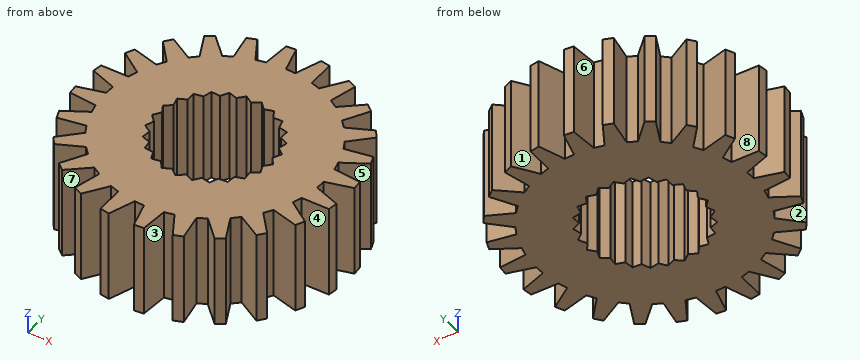
```python
from build123d import *

# Parameters (mm, degrees)
F1_DEPTH = 5.08


# Not quite as in the source:
# - ends of sketch curves that miss each other by under 0.0002 mm in the source are joined


with BuildPart() as f1:
    # F0 (on Top) → F1 (new body)
    with BuildSketch(Plane.XY):
        with BuildLine():
            Line((1.0386822, 7.3975722), (0.5233416, 5.9817))
            ThreePointArc((0.5233416, 5.9817), (0.261920534, 5.9988447577), (0, 6.00456))
            Line((0, 6.00456), (-0.3899662, 7.4599546))
            Line((-0.3899662, 7.4599546), (-0.911352, 7.4143362))
            Line((-0.911352, 7.4143362), (-1.04267, 5.9133486))
            ThreePointArc((-1.04267, 5.9133486), (-1.2996201412, 5.8622289517), (-1.5540978425, 5.79995868))
            Line((-1.5540978425, 5.79995868), (-2.307463, 7.1048372))
            Line((-2.307463, 7.1048372), (-2.7992832, 6.925818))
            Line((-2.7992832, 6.925818), (-2.5376378, 5.4419754))
            ThreePointArc((-2.5376378, 5.4419754), (-2.7726007409, 5.3261079528), (-3.0022844594, 5.2000989239))
            Line((-3.0022844594, 5.2000989239), (-4.0677084, 6.2655196))
            Line((-4.0677084, 6.2655196), (-4.496435, 5.965317))
            Line((-4.496435, 5.965317), (-3.859657, 4.5997622))
            ThreePointArc((-3.859657, 4.5997622), (-4.0566214385, 4.4270264624), (-4.245865094, 4.245865094))
            Line((-4.245865094, 4.245865094), (-5.5507382, 4.999228))
            Line((-5.5507382, 4.999228), (-5.8871612, 4.598289))
            Line((-5.8871612, 4.598289), (-4.9186338, 3.4440622))
            ThreePointArc((-4.9186338, 3.4440622), (-5.0641936548, 3.2262491255), (-5.2000989239, 3.0022844594))
            Line((-5.2000989239, 3.0022844594), (-6.6554858, 3.3922462))
            Line((-6.6554858, 3.3922462), (-6.876669, 2.9179012))
            Line((-6.876669, 2.9179012), (-5.6424322, 2.0536916))
            ThreePointArc((-5.6424322, 2.0536916), (-5.7266481207, 1.8056140494), (-5.79995868, 1.5540978425))
            Line((-5.79995868, 1.5540978425), (-7.306691, 1.554099))
            Line((-7.306691, 1.554099), (-7.3975722, 1.0386568))
            Line((-7.3975722, 1.0386568), (-5.9817, 0.5233416))
            ThreePointArc((-5.9817, 0.5233416), (-5.9988447577, 0.261920534), (-6.00456, 0))
            Line((-6.00456, 0), (-7.4599546, -0.3899662))
            Line((-7.4599546, -0.3899662), (-7.4143362, -0.911352))
            Line((-7.4143362, -0.911352), (-5.9133232, -1.04267))
            ThreePointArc((-5.9133232, -1.04267), (-5.8622284744, -1.2996222942), (-5.79995868, -1.5540978425))
            Line((-5.79995868, -1.5540978425), (-7.1048372, -2.307463))
            Line((-7.1048372, -2.307463), (-6.925818, -2.7992832))
            Line((-6.925818, -2.7992832), (-5.4419754, -2.5376378))
            ThreePointArc((-5.4419754, -2.5376378), (-5.3261079528, -2.7726007409), (-5.2000989239, -3.0022844594))
            Line((-5.2000989239, -3.0022844594), (-6.2655196, -4.0677084))
            Line((-6.2655196, -4.0677084), (-5.965317, -4.496435))
            Line((-5.965317, -4.496435), (-4.5997622, -3.859657))
            ThreePointArc((-4.5997622, -3.859657), (-4.4270264624, -4.0566214385), (-4.245865094, -4.245865094))
            Line((-4.245865094, -4.245865094), (-4.999228, -5.5507382))
            Line((-4.999228, -5.5507382), (-4.598289, -5.8871612))
            Line((-4.598289, -5.8871612), (-3.4440622, -4.9186592))
            ThreePointArc((-3.4440622, -4.9186592), (-3.2262429819, -5.0641975688), (-3.0022844594, -5.2000989239))
            Line((-3.0022844594, -5.2000989239), (-3.3922462, -6.6554858))
            Line((-3.3922462, -6.6554858), (-2.9179012, -6.8766944))
            Line((-2.9179012, -6.8766944), (-2.0536662, -5.6424322))
            ThreePointArc((-2.0536662, -5.6424322), (-1.8056026676, -5.7266517094), (-1.5540978425, -5.79995868))
            Line((-1.5540978425, -5.79995868), (-1.554099, -7.306691))
            Line((-1.554099, -7.306691), (-1.0386568, -7.3975722))
            Line((-1.0386568, -7.3975722), (-0.5233162, -5.9817))
            ThreePointArc((-0.5233162, -5.9817), (-0.2619078943, -5.9988453096), (0, -6.00456))
            Line((0, -6.00456), (0.3899662, -7.4599546))
            Line((0.3899662, -7.4599546), (0.9113774, -7.4143362))
            Line((0.9113774, -7.4143362), (1.0426954, -5.9133486))
            ThreePointArc((1.0426954, -5.9133486), (1.2996323518, -5.8622262447), (1.5540978425, -5.79995868))
            Line((1.5540978425, -5.79995868), (2.307463, -7.1048372))
            Line((2.307463, -7.1048372), (2.7992832, -6.925818))
            Line((2.7992832, -6.925818), (2.5376378, -5.4419754))
            ThreePointArc((2.5376378, -5.4419754), (2.7726007409, -5.3261079528), (3.0022844594, -5.2000989239))
            Line((3.0022844594, -5.2000989239), (4.0677084, -6.2655196))
            Line((4.0677084, -6.2655196), (4.496435, -5.965317))
            Line((4.496435, -5.965317), (3.859657, -4.5997622))
            ThreePointArc((3.859657, -4.5997622), (4.0566214385, -4.4270264624), (4.245865094, -4.245865094))
            Line((4.245865094, -4.245865094), (5.5507382, -4.999228))
            Line((5.5507382, -4.999228), (5.8871612, -4.598289))
            Line((5.8871612, -4.598289), (4.9186592, -3.4440622))
            ThreePointArc((4.9186592, -3.4440622), (5.0642009806, -3.2262376264), (5.2001052739, -3.0022734609))
            Line((5.2001052739, -3.0022734609), (6.6555112, -3.3922462))
            Line((6.6555112, -3.3922462), (6.8766944, -2.9179012))
            Line((6.8766944, -2.9179012), (5.6424576, -2.0536916))
            ThreePointArc((5.6424576, -2.0536916), (5.7266494269, -1.8056099067), (5.79995868, -1.5540978425))
            Line((5.79995868, -1.5540978425), (7.306691, -1.554099))
            Line((7.306691, -1.554099), (7.3975722, -1.0386568))
            Line((7.3975722, -1.0386568), (5.9817254, -0.5233416))
            ThreePointArc((5.9817254, -0.5233416), (5.998844806, -0.2619194281), (6.00456, 0))
            Line((6.00456, 0), (7.4599546, 0.3899662))
            Line((7.4599546, 0.3899662), (7.4143362, 0.911352))
            Line((7.4143362, 0.911352), (5.9133486, 1.04267))
            ThreePointArc((5.9133486, 1.04267), (5.8622289517, 1.2996201412), (5.79995868, 1.5540978425))
            Line((5.79995868, 1.5540978425), (7.1048372, 2.307463))
            Line((7.1048372, 2.307463), (6.925818, 2.7992832))
            Line((6.925818, 2.7992832), (5.4419754, 2.5376378))
            ThreePointArc((5.4419754, 2.5376378), (5.3261108849, 2.7725951084), (5.2001052739, 3.0022734609))
            Line((5.2001052739, 3.0022734609), (6.2655196, 4.0677084))
            Line((6.2655196, 4.0677084), (5.9653424, 4.496435))
            Line((5.9653424, 4.496435), (4.5997622, 3.859657))
            ThreePointArc((4.5997622, 3.859657), (4.4270264624, 4.0566214385), (4.245865094, 4.245865094))
            Line((4.245865094, 4.245865094), (4.999228, 5.5507382))
            Line((4.999228, 5.5507382), (4.5983144, 5.8871612))
            Line((4.5983144, 5.8871612), (3.4440876, 4.9186592))
            ThreePointArc((3.4440876, 4.9186592), (3.2262517559, 5.0641919791), (3.0022844594, 5.2000989239))
            Line((3.0022844594, 5.2000989239), (3.3922462, 6.6554858))
            Line((3.3922462, 6.6554858), (2.9179012, 6.8766944))
            Line((2.9179012, 6.8766944), (2.0536916, 5.6424322))
            ThreePointArc((2.0536916, 5.6424322), (1.8056140494, 5.7266481207), (1.5540978425, 5.79995868))
            Line((1.5540978425, 5.79995868), (1.554099, 7.306691))
            Line((1.554099, 7.306691), (1.0386822, 7.3975722))
        make_face()
        Polygon((-1.2318492, 3.1113222), (-0.7605522, 2.9622242), (-0.4194048, 3.319907), (0, 3.0583124), (0.4194048, 3.319907), (0.7605776, 2.9622242), (1.2318492, 3.1113222), (1.4733524, 2.6800048), (1.9668998, 2.7072082), (2.0935442, 2.2294088), (2.5783794, 2.1330158), (2.5822148, 1.6387318), (3.0278324, 1.4247876), (2.9086302, 0.9450578), (3.2870394, 0.6270244), (3.0522672, 0.192024), (3.3396936, -0.2101088), (3.0041342, -0.5730748), (3.1825184, -1.0340594), (2.7672284, -1.3021564), (2.825369, -1.7930368), (2.3564596, -1.9494246), (2.290699, -2.4393398), (1.7976342, -2.474214), (1.6120872, -2.9323792), (1.1258296, -2.84353), (0.8322056, -3.241167), (0.3833114, -3.0341824), (0, -3.3462976), (-0.3833114, -3.0341824), (-0.8321802, -3.241167), (-1.1258296, -2.84353), (-1.6120872, -2.9323792), (-1.7976088, -2.474214), (-2.290699, -2.4393398), (-2.3564596, -1.9494246), (-2.825369, -1.7930368), (-2.7672284, -1.3021564), (-3.1825184, -1.0340594), (-3.0041342, -0.5730748), (-3.3396936, -0.2101088), (-3.0522672, 0.192024), (-3.287014, 0.6270244), (-2.9086048, 0.9450578), (-3.027807, 1.4247876), (-2.5822148, 1.6387318), (-2.578354, 2.1330158), (-2.0935442, 2.2294088), (-1.9668998, 2.7072082), (-1.4733524, 2.6800048), align=None, mode=Mode.SUBTRACT)
    extrude(amount=F1_DEPTH)


solid = f1.part
```
Could you check a few things on this model? Use its own coordinates, in mm. Face numbers are marked on the shaded views. A direction names the side the tool comes from. Round coordinates to 2 decimals unless told otherwise and drop trailing zeros. Put each result on its own line as item: value.
Q1. Thinking about a two-plate mould opening in Y: for the marked faces 1, 2, 3 and 4, which applies, pulls with the +Y half, pulls with the -Y half, needs draft (parallel to the pull), parting line crosses it, or undercut?
Checks:
face 1: pulls with the +Y half
face 2: undercut
face 3: pulls with the -Y half
face 4: undercut
Q2. Which directions (+Z, -Z, +X, -X, +Y, -Y) give clear straight access to the entire face, cutting with the end or side of a thin tool? Please do the marked faces 5, 6, 7 and 8.
Checks:
face 5: +Z, -Z, +X
face 6: +Z, -Z, +Y
face 7: +Z, -Z, -Y
face 8: +Z, -Z, -X
Q3. For pin 1 Ø0.5 at (x, z) = (-6.5, 2.5) entering from +Y; pin 2 Ø2 at (y, z) = (-4, 1.5) entering from +X; pin 3 Ø1.5 at (y, z) = (4.5, 2.5) entering from +X, each with a flat end and sliding along its axis, tell me the tip position at first contact or that it passes through.
Checks:
pin 1: y = 3.39
pin 2: x = 6.84
pin 3: x = 6.27
Q4. Please list where these lines run through material, in increasing order: line 1 (Y direction, x = 5.5, z = 2.2); line 2 (Y direction, x = -6.5, z = 4.1); line 3 (Y direction, x = 6.75, z = 0.75). Write a range as from..to.
Checks:
line 1: -4.97..-4.14, -3.08..2.55, 3.3..4.28
line 2: -2.72..-1.96, -0.99..-0.13, 0.71..1.55, 2.65..3.35
line 3: -3.19..-2.83, -1.55..-0.8, 0.2..0.97, 2.1..2.77
